Read the model definition and answer for the solid it produces. Units are mm, in the model's axes. A direction names the side the tool comes from. Coordinates: 2 decimals unless noted, no trailing zeros. Loops run counter-clockwise (first coordinate to the right, second up) from the corner with the lowest first, then second, coordinate; pieces in that order, holes last. Notation, with made-up numbers: M 55.5,12.25 L 110.5,12.25 A23 cw 110.5,41.25 Z; hole C 47,41 d9. An arc over 180 degrees is marked long. Put each result on its own line as item: value.
from build123d import *

# Parameters (mm, degrees)
F1_DEPTH  = 9
F2_W      = 7
F2_H      = 42
F3_DEPTH  = 21
F5_DEPTH  = 25
F7_DEPTH  = 30
F8_DEPTH  = 21
F9_R      = 7.5
F10_DEPTH = 30


with BuildPart() as f1:
    # F0 (on Top) → F1 (new body)
    with BuildSketch(Plane.XY):
        Polygon((15, 30), (-15, 30), (-15, -21), (-6, -30), (6, -30), (15, -21), align=None)
    extrude(amount=F1_DEPTH)

    # F2 (on face) → F3 (join)
    with BuildSketch(Plane.XY.offset(9)):
        with Locations((0.25, -9)):
            Rectangle(F2_W, F2_H)
    extrude(amount=F3_DEPTH)

    # F4 (on face) → F5 (cut)
    with BuildSketch(Plane(origin=(-3.25, 0, 0), x_dir=(0, -1, 0), z_dir=(-1, 0, 0))):
        Polygon((30, 30), (-7.5259371102, 30), (30, 11.2370314449), align=None)
    extrude(amount=-F5_DEPTH, mode=Mode.SUBTRACT)

    # F0 (on Top) → F7 (join)
    with BuildSketch(Plane.XY):
        with BuildLine():
            ThreePointArc((15, 30), (0, 45), (-15, 30))
            Line((-15, 30), (15, 30))
        make_face()
    extrude(amount=F7_DEPTH)

    # F6 (on face) → F8 (join)
    with BuildSketch(Plane.XY.offset(9)):
        Polygon((3.75, 12), (15, 12), (15, 30), (-15, 30), (-15, 12), (-3.25, 12), align=None)
    extrude(amount=F8_DEPTH)

    # F9 (on face) → F10 (cut)
    with BuildSketch(Plane.XY.offset(30)):
        with Locations((0, 30)):
            Circle(F9_R)
    extrude(amount=-F10_DEPTH, mode=Mode.SUBTRACT)


solid = f1.part
1) Find section D-D, the plane z = 10.25. Write down the section's boundary in (x, y).
Answer list:
outline: M -15,12 L -3.25,12 L -3.25,-30 L 3.75,-30 L 3.75,12 L 15,12 L 15,30 A15 ccw -15,30 Z; hole C 0,30 d15
2) Determine the mould class of faces 1 (the cylindrical face through (-1.63, 22.68, 15.21)), 2 (the cylindrical face through (0, 45, 15)), 3 (the flat face through (-11, -25, 4)) for opening direction X: released by +X, released by -X, zero draft, split by the parting line, or undercut.
Answer list:
face 1: undercut
face 2: split by the parting line
face 3: released by -X
3) Find section A-A, the plane x = 0. Write down the section's boundary in (y, z).
Answer list:
outline: M -30,0 L 22.5,0 L 22.5,30 L 7.53,30 L -30,11.24 Z; M 37.5,0 L 45,0 L 45,30 L 37.5,30 Z
4) Find section B-B, the plane z = 5.25. Write down the section's boundary in (x, y), plus the area to 3 significant figures.
Answer list:
outline: M -15,-21 L -6,-30 L 6,-30 L 15,-21 L 15,30 A15 ccw -15,30 Z; hole C 0,30 d15
area: 1,900 mm^2
5) Straight lines are drawn through the part: line 1 (Y direction, x = 0, z = 7.5); line 2 (X direction, y = -6, z = 22.5); line 3 (Y direction, x = 0, z = 16.25). For each, find the intervals that lie inside material, in ascending order. Write a range as [from, to].
Answer list:
line 1: y = [-30, 22.5], [37.5, 45]
line 2: x = [-3.25, 3.75]
line 3: y = [-19.97, 22.5], [37.5, 45]
6) Find section C-C, the plane y = 31. Write down the section's boundary in (x, z).
Answer list:
outline: M -14.97,0 L -7.43,0 L -7.43,30 L -14.97,30 Z; M 7.43,0 L 14.97,0 L 14.97,30 L 7.43,30 Z
7) Given pin 1 Ø6 at (x, z) = (3.5, 22.5) entering from -Y; pin 2 Ø9 at (x, z) = (8.5, 24) entering from -Y; pin 3 Ø1 at (y, z) = (-22.5, 6.5) entering from +X, each flat-ended and moving along its own axis, determine where each tip first touches the part or whether it passes through.
Answer list:
pin 1: stops at y = -13.47
pin 2: stops at y = 12
pin 3: stops at x = 14
8) Which of the six approach directions +Z, -Z, +X, -X, +Y, -Y give full straight-line access (tool end or side, diameter ignored) to faces 4 (the flat face through (-15, 11, 8)), 5 (the flat face through (-9, -9, 9)), 6 (the flat face through (9, 12, 19))?
Answer list:
face 4: +Z, -Z, -X, +Y, -Y
face 5: +Z, -X, -Y
face 6: +Z, +X, -Y
